Part model, mm, in its own coordinate system. Face numbers are marked on the shaded views. A direction names the side the tool comes from. Coordinates: 2 decimals unless noted, no trailing zeros. Order: outer loops, then holes, each group sorted by start corner. A loop starts at its lowest first (then second) coordinate and runs counter-clockwise, first axis right, second up.
1) Cut at C-C (z = 11.25). List the corners of the cut face in (x, y).
2) Cut at D-D (y = -2.25). List the corners of the cut face in (x, z), and give its area (3 significant figures).
3) Tool access for the marked faces 4 and 5: list every direction of +Z, -Z, +X, -X, +Y, -Y with a clear straight run to the whole face (end or side of a thin tool).
4) Cut at B-B (y = -0.5). List the corners of the cut face in (x, z), and give its area (3 significant figures).
5) Pin check, flat tips, straight feed: pin 1 Ø1 at (y, z) = (3, 19.5) entering from -X; pin 2 Ø1.8 at (x, y) = (1.5, -1.5) entering from +Z; pin 3 Ø3 at (y, z) = (-2, 15) entering from +X. Stop position of each tip, or through.
6) Wall check: L1, parallel to Y at x = 0, z = 7.25; L2, parallel to Z at x = -2.25, y = -1; L3, parallel to Y at x = -1.5, z = 2.5. Give the ranges that are in metal, low to high.
7) Mould opens along X. For the marked faces 1, 2 and 3 say: +X half, -X half, draft (parallel to the pull), parting line (faces both ways), or undercut.
8) Cut at A-A (x = 0). List the corners of the cut face in (y, z), and give its area (3 significant figures).
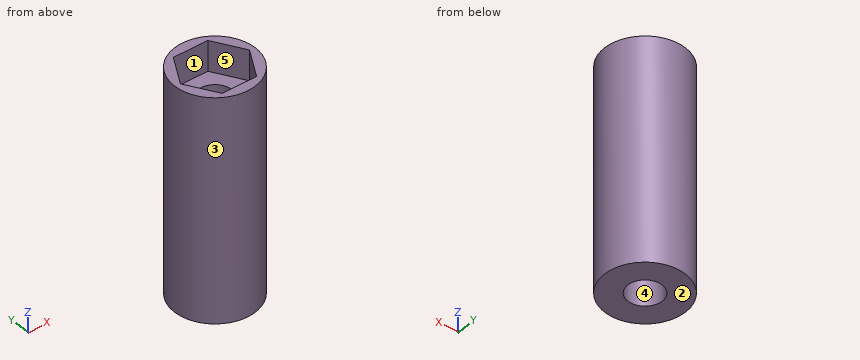
```python
from build123d import *

# Parameters (mm, degrees)
SKETCH001_R     = 4
PAD001_DEPTH    = 22
POCKET_DEPTH    = 3
SKETCH002_R     = 1.7
POCKET001_DEPTH = 30


with BuildPart() as part:
    # Sketch001 → Pad001 (new body)
    with BuildSketch(Plane.XY):
        Circle(SKETCH001_R)
    extrude(amount=PAD001_DEPTH)

    # Sketch → Pocket (cut)
    with BuildSketch(Plane.XY.offset(22)):
        Polygon((-1.732051, 3), (1.732051, 3), (3.464102, 0), (1.732051, -3), (-1.732051, -3), (-3.464102, 0), align=None)
    extrude(amount=-POCKET_DEPTH, mode=Mode.SUBTRACT)

    # Sketch002 → Pocket001 (cut)
    with BuildSketch(Plane(origin=(0, 0, 0), x_dir=(1, 0, 0), z_dir=(0, 0, -1))):
        Circle(SKETCH002_R)
    extrude(amount=-POCKET001_DEPTH, mode=Mode.SUBTRACT)


solid = part.part
```
Geometry check:
1. outline: circle Ø8 at (0, 0); hole circle Ø3.4 at (0, 0)
2. outline: (-3.31, 0) - (3.31, 0) - (3.31, 22) - (2.17, 22) - (2.17, 19) - (-2.17, 19) - (-2.17, 22) - (-3.31, 22) - close
2. area: 133 mm2
3. face 4: +Z, -Z
3. face 5: +Z
4. outline: (-3.97, 0) - (-1.62, 0) - (-1.62, 19) - (-3.18, 19) - (-3.18, 22) - (-3.97, 22) - close; (1.62, 0) - (3.97, 0) - (3.97, 22) - (3.18, 22) - (3.18, 19) - (1.62, 19) - close
4. area: 93.8 mm2
5. pin 1: stops at x = -3.12
5. pin 2: stops at z = 19
5. pin 3: stops at x = 3.97
6. L1: y = -4 to -1.7, 1.7 to 4
6. L2: z = 0 to 19
6. L3: y = -3.71 to -0.8, 0.8 to 3.71
7. face 1: undercut
7. face 2: draft
7. face 3: parting line
8. outline: (-4, 0) - (-1.7, 0) - (-1.7, 19) - (-3, 19) - (-3, 22) - (-4, 22) - close; (1.7, 0) - (4, 0) - (4, 22) - (3, 22) - (3, 19) - (1.7, 19) - close
8. area: 93.4 mm2
